from build123d import *

# Parameters (mm, degrees)
SKETCH1_R           = 2.5
BOSS_EXTRUDE1_DEPTH = 5
BOSS_EXTRUDE2_START = -5
BOSS_EXTRUDE2_DEPTH = 5
SKETCH8_W           = 9.009618943
SKETCH8_H           = 15
BOSS_EXTRUDE3_DEPTH = 20
SKETCH1_3_R         = 6.5
CUT_EXTRUDE1_DEPTH  = 89.888975736
FILLET1_R           = 6
BOSS_EXTRUDE4_START = 1
SKETCH1_4_R         = 6.5
SKETCH1_4_R_2       = 2.5
BOSS_EXTRUDE4_DEPTH = 1


with BuildPart() as part:
    # Sketch1 → Boss-Extrude1 (new body)
    with BuildSketch(Plane(origin=(0, 0, 0), x_dir=(0, 1, 0), z_dir=(0, 0, 1))):
        with BuildLine():
            ThreePointArc((23.466233734, -14.338266086), (27.5, 0), (23.466233734, 14.338266086))
            ThreePointArc((23.466233734, 14.338266086), (24.04163056, 24.04163056), (14.338266086, 23.466233734))
            ThreePointArc((14.338266086, 23.466233734), (0, 27.5), (-14.338266086, 23.466233734))
            ThreePointArc((-14.338266086, 23.466233734), (-24.04163056, 24.04163056), (-23.466233734, 14.338266086))
            ThreePointArc((-23.466233734, 14.338266086), (-27.5, 0), (-23.466233734, -14.338266086))
            ThreePointArc((-23.466233734, -14.338266086), (-24.04163056, -24.04163056), (-14.338266086, -23.466233734))
            ThreePointArc((-14.338266086, -23.466233734), (0, -27.5), (14.338266086, -23.466233734))
            ThreePointArc((14.338266086, -23.466233734), (24.04163056, -24.04163056), (23.466233734, -14.338266086))
        make_face()
        with Locations(Location((-19.445436483, 19.445436483, 0), (0, 0, 270))):
            Circle(SKETCH1_R, mode=Mode.SUBTRACT)
        with Locations(Location((19.445436483, 19.445436483, 0), (0, 0, 270))):
            Circle(SKETCH1_R, mode=Mode.SUBTRACT)
        with Locations(Location((19.445436483, -19.445436483, 0), (0, 0, 270))):
            Circle(SKETCH1_R, mode=Mode.SUBTRACT)
        with Locations(Location((-19.445436483, -19.445436483, 0), (0, 0, 270))):
            Circle(SKETCH1_R, mode=Mode.SUBTRACT)
    extrude(amount=-BOSS_EXTRUDE1_DEPTH)

    # Sketch5 → Revolve1 (revolve)
    with BuildSketch(Plane.YZ, mode=Mode.PRIVATE) as revolve1_sk:
        Polygon((0, 0), (24, 0), (13.5, 9), (0, 9), align=None)
    revolve(revolve1_sk.sketch.rotate(Axis((0, 0, 9), (0, 0, -1)), 180), axis=Axis((0, 0, 9), (0, 0, -1)))

    # Sketch6 → Boss-Extrude2 (add)
    with BuildSketch(Plane.YX.offset(5).offset(BOSS_EXTRUDE2_START)):
        with BuildLine():
            ThreePointArc((0, 37), (-9.854658782, 33.30865599), (-14.859059475, 24.051426706))
            ThreePointArc((-14.859059475, 24.051426706), (-14.589838885, 23.766683059), (-14.338266086, 23.466233734))
            ThreePointArc((-14.338266086, 23.466233734), (-7.447434871, 26.472357542), (0, 27.5))
            Line((0, 27.5), (0, 37))
        make_face()
        with BuildLine():
            ThreePointArc((14.859059475, 24.051426706), (9.854658782, 33.30865599), (0, 37))
            Line((0, 37), (0, 27.5))
            ThreePointArc((0, 27.5), (7.447434871, 26.472357542), (14.338266086, 23.466233734))
            ThreePointArc((14.338266086, 23.466233734), (14.589838885, 23.766683059), (14.859059475, 24.051426706))
        make_face()
        with BuildLine():
            Line((-14.626824069, 37), (-24.04163056, 24.04163056))
            ThreePointArc((-24.04163056, 24.04163056), (-19.452370805, 25.945432784), (-14.859059475, 24.051426706))
            ThreePointArc((-14.859059475, 24.051426706), (-9.854658782, 33.30865599), (0, 37))
            Line((0, 37), (-14.626824069, 37))
        make_face()
        with BuildLine():
            ThreePointArc((-14.338266086, 23.466233734), (-14.589838885, 23.766683059), (-14.859059475, 24.051426706))
            ThreePointArc((-14.859059475, 24.051426706), (-1.028131286, 7.035276613), (15, 22))
            ThreePointArc((15, 22), (14.964723387, 23.028131286), (14.859059475, 24.051426706))
            ThreePointArc((14.859059475, 24.051426706), (14.589838885, 23.766683059), (14.338266086, 23.466233734))
            ThreePointArc((14.338266086, 23.466233734), (7.447434871, 26.472357542), (0, 27.5))
            ThreePointArc((0, 27.5), (-7.447434871, 26.472357542), (-14.338266086, 23.466233734))
        make_face()
    extrude(amount=BOSS_EXTRUDE2_DEPTH)

    # Sketch7 → Revolve2 (revolve)
    with BuildSketch(Plane(origin=(0, 0, 0), x_dir=(-1, 0, 0), z_dir=(0, 1, 0)), mode=Mode.PRIVATE) as revolve2_sk:
        Polygon((-22, 0), (-22, 76), (-27, 76), (-27, 66), (-28.5, 66), (-28.5, 61), (-29.5, 61), (-29.5, 32), (-34.5, 32), (-34.5, 31), (-37, 31), (-37, 0), align=None)
    revolve(revolve2_sk.sketch.rotate(Axis((22, 0, 0), (0, 0, 1)), 180), axis=Axis((22, 0, 0), (0, 0, 1)))

    # Sketch8 → Boss-Extrude3 (add)
    with BuildSketch(Plane.XY.offset(9)):
        with Locations((4.504809472, 0)):
            Rectangle(SKETCH8_W, SKETCH8_H)
    extrude(amount=BOSS_EXTRUDE3_DEPTH)

    # Sketch1<3> → Cut-Extrude1 (cut, through all)
    with BuildSketch(Plane(origin=(0, 0, 0), x_dir=(0, 1, 0), z_dir=(0, 0, 1))):
        with Locations((19.445436483, 19.445436483)):
            Circle(SKETCH1_3_R)
        with Locations((-19.445436483, 19.445436483)):
            Circle(SKETCH1_3_R)
        with Locations((-19.445436483, -19.445436483)):
            Circle(SKETCH1_3_R)
        with Locations((19.445436483, -19.445436483)):
            Circle(SKETCH1_3_R)
    extrude(amount=CUT_EXTRUDE1_DEPTH, mode=Mode.SUBTRACT)

    # Fillet1
    fillet1_edges = [part.edges().sort_by_distance(p)[0] for p in [
        (37, -14.626824069, -2.5),
    ]]
    fillet(fillet1_edges, radius=FILLET1_R)

    # Sketch1<4> → Boss-Extrude4 (add)
    # profile 1 of 4: a face of its own
    with BuildSketch(Plane(origin=(0, 0, 0), x_dir=(0, 1, 0), z_dir=(0, 0, 1)).offset(BOSS_EXTRUDE4_START)):
        with Locations((19.445436483, 19.445436483)):
            Circle(SKETCH1_4_R)
        with Locations(Location((19.445436483, 19.445436483, 0), (0, 0, 270))):
            Circle(SKETCH1_4_R_2, mode=Mode.SUBTRACT)
    # profile 2 of 4: a face of its own
    with BuildSketch(Plane(origin=(0, 0, 0), x_dir=(0, 1, 0), z_dir=(0, 0, 1)).offset(BOSS_EXTRUDE4_START)):
        with Locations((19.445436483, -19.445436483)):
            Circle(SKETCH1_4_R)
        with Locations(Location((19.445436483, -19.445436483, 0), (0, 0, 270))):
            Circle(SKETCH1_4_R_2, mode=Mode.SUBTRACT)
    # profile 3 of 4: a face of its own
    with BuildSketch(Plane(origin=(0, 0, 0), x_dir=(0, 1, 0), z_dir=(0, 0, 1)).offset(BOSS_EXTRUDE4_START)):
        with Locations((-19.445436483, 19.445436483)):
            Circle(SKETCH1_4_R)
        with Locations(Location((-19.445436483, 19.445436483, 0), (0, 0, 270))):
            Circle(SKETCH1_4_R_2, mode=Mode.SUBTRACT)
    # profile 4 of 4: a face of its own
    with BuildSketch(Plane(origin=(0, 0, 0), x_dir=(0, 1, 0), z_dir=(0, 0, 1)).offset(BOSS_EXTRUDE4_START)):
        with Locations((-19.445436483, -19.445436483)):
            Circle(SKETCH1_4_R)
        with Locations(Location((-19.445436483, -19.445436483, 0), (0, 0, 270))):
            Circle(SKETCH1_4_R_2, mode=Mode.SUBTRACT)
    extrude(amount=-BOSS_EXTRUDE4_DEPTH)


solid = part.part
Build history of the part. All positions in model axes, mm. A direction names the side the tool comes from. Coordinates: 2 decimals unless noted, no trailing zeros. Order: outer loops, then holes, each group sorted by start corner. A loop starts at its lowest first (then second) coordinate and runs counter-clockwise, first axis right, second up. Notation, with made-up numbers: (61.5, 62.5) - (108.5, 62.5) arc R19 cw to (108.5, 82.5) - close; hole circle Ø11 at (60, 21). An arc over 180 degrees is marked (long way). Write item = value, one per line. Start each with the question number.
1) 3-axis set-ups, long thin cutter, end or side, ignore diameter. For faces 1 (the face through (20.384, 13.014, 15.79)), 2 (the face through (28.494, -0.286, 63.465)), 3 (the face through (-19.5, -16.6, 1)), 4 (the face through (-14.9, 14.8, 1.6)), 5 (the face through (0, -25, 0)): which of +Z, -Z, +X, -X, +Y, -Y reach the whole face in a straight line?
2) Wall check: line 1 along Z through (x, y) = (29, -16); line 2 along Z through (x, y) = (11.5, 1); line 3 along X through (y, z) = (12, 19). Give the ranges that are in metal, low to high. Write a range as from..to.
3) Saw through at B-B on z = 49. Write the cut outline in (x, y), then the cut area to 3 significant figures.
4) Saw through at A-A on z = 22.5. Write the cut outline in (x, y), then the cut area to 3 significant figures.
5) Flat gauge pins, fed straight in: pin 1 Ø4 at (x, z) = (-1.5, 20) entering from +Y; pin 2 Ø4 at (x, y) = (29.5, -13.5) entering from +Z; pin 3 Ø5 at (x, z) = (-8, 10.5) entering from -Y. Where does each tip first touch, or does it go through?
From the geometry:
q1.face_1 = +Z, +Y
q1.face_2 = +Z
q1.face_3 = +Z, -X, -Y
q1.face_4 = +Z, -X, +Y
q1.face_5 = +Z, -Y
q2.line_1 = -5..0
q2.line_2 = -5..32
q2.line_3 = 13..31
q3.outline = circle Ø15 at (22, 0)
q3.area = 177 mm^2
q4.outline = (0, -7.5) - (9.01, -7.5) arc R15 ccw to (16.18, -13.83) arc R6.5 cw to (24.05, -14.86) arc R15 ccw to (24.05, 14.86) arc R6.5 cw to (16.18, 13.83) arc R15 ccw to (9.01, 7.5) - (0, 7.5) - close
q4.area = 801 mm^2
q5.pin_1 = 7.5
q5.pin_2 = 31
q5.pin_3 = -12.61
